Here's how the part is built. I have some questions about the finished solid (model axes, mm). A direction names the side the tool comes from. Coordinates: 2 decimals unless noted, no trailing zeros. Write each loop counter-clockwise with the first axis right and the second up, starting at its lowest first coordinate (ties: lowest second). Pieces come first, ordered by that corner, then holes. Notation, with made-up numbers: M -26.75,31 L -14.75,31 A32 ccw -14.75,60 Z; hole C -32,12 d9. An arc over 180 degrees is marked long. Use a Markdown table: item, result.
```python
from build123d import *

# Parameters (mm, degrees)
SKETCH1_W             = 10
SKETCH1_H             = 10.5
CUT_EXTRUDE1_DEPTH    = 11
CIRPATTERN1_COUNT     = 11
SKETCH3_R             = 12.5
BOSS_EXTRUDE1_DEPTH   = 10
CUT_EXTRUDE2_DEPTH    = 21
M2_TAPPED_HOLE1_D     = 1.6
M2_TAPPED_HOLE1_DEPTH = 9.8


with BuildPart() as part:
    # Sketch1 → Revolve1 (revolve)
    with BuildSketch(Plane(origin=(0, 0, 0), x_dir=(0, 0, -1), z_dir=(1, 0, 0))):
        with Locations((5, 5.25)):
            Rectangle(SKETCH1_W, SKETCH1_H)
    revolve(axis=Axis((0, 0, 0), (0, 0, -1)))

    # Sketch2 → Cut-Extrude1 (cut, through all)
    with BuildSketch(Plane.XY):
        with BuildLine():
            ThreePointArc((-0.824529961, 7.076123681), (0, 7.124), (0.824529961, 7.076123681))
            ThreePointArc((0.824529961, 7.076123681), (1.228997776, 8.871328839), (2.467796901, 10.232112622))
            ThreePointArc((2.467796901, 10.232112622), (0, 10.5255), (-2.467796901, 10.232112622))
            ThreePointArc((-2.467796901, 10.232112622), (-1.228997776, 8.871328839), (-0.824529961, 7.076123681))
        make_face()
    cut_extrude1 = extrude(amount=-CUT_EXTRUDE1_DEPTH, mode=Mode.SUBTRACT)

    # CirPattern1: Cut-Extrude1 ×11 about axis
    cirpattern1_axis = Axis((0, 0, 0), (0, 0, 1))
    for i in range(1, CIRPATTERN1_COUNT):
        add(cut_extrude1.rotate(cirpattern1_axis, i * 360 / CIRPATTERN1_COUNT), mode=Mode.SUBTRACT)

    # Sketch3 → Boss-Extrude1 (add)
    with BuildSketch(Plane.XY):
        Circle(SKETCH3_R)
    extrude(amount=BOSS_EXTRUDE1_DEPTH)

    # Sketch4 → Cut-Extrude2 (cut, through all)
    with BuildSketch(Plane.XY.offset(10)):
        with BuildLine():
            Line((2.7, 1.622498074), (2.7, -1.622498074))
            ThreePointArc((2.7, -1.622498074), (-3.15, 0), (2.7, 1.622498074))
        make_face()
    extrude(amount=-CUT_EXTRUDE2_DEPTH, mode=Mode.SUBTRACT)

    # M2 Tapped Hole1
    with Locations(Plane(origin=(12.5, 0, 0), x_dir=(0, 0, -1), z_dir=(1, 0, 0))):
        with Locations((-5, 0)):
            Hole(M2_TAPPED_HOLE1_D / 2, depth=M2_TAPPED_HOLE1_DEPTH)


solid = part.part
```
1. Will these pins go through, and if not, where does the flat tip stop? pin 1 Ø4 at (x, y) = (0, 0) entering from -Z; pin 2 Ø3 at (x, z) = (5, 7) entering from -Y; pin 3 Ø10 at (y, z) = (-9.5, 4) entering from -X; pin 4 Ø5 at (x, z) = (-8.5, 0.5) entering from +Y.
Answers follow:
| item | result |
|---|---|
| pin 1 | passes through |
| pin 2 | stops at y = -12 |
| pin 3 | stops at x = -11.66 |
| pin 4 | stops at y = 10.97 |
2. Suppose I cut it at C-C on z = 5. Write out the boundary of the cut face in (x, y).
Answers follow:
| item | result |
|---|---|
| outline | M 2.7,-1.62 A3.15 cw long 2.7,1.62 L 2.7,0.8 L 12.47,0.8 A12.5 ccw long 12.47,-0.8 L 2.7,-0.8 Z |
3. Suppose I cut it at B-B on y = -6. Write out the boundary of the cut face in (x, z).
Answers follow:
| item | result |
|---|---|
| outline | M -10.97,0 L -5.5,0 L -5.5,-10 L 5.5,-10 L 5.5,0 L 10.97,0 L 10.97,10 L -10.97,10 Z |
4. Which directions (+Z, -Z, +X, -X, +Y, -Y) give clear straight access to the entire face, cutting with the end or side of a thin tool? Please do faces 1 (the face through (9.55, -4.36, -5.07)), 2 (the face through (10.392, 1.502, -5.07)).
Answers follow:
| item | result |
|---|---|
| face 1 | -Z, +X, -Y |
| face 2 | -Z, +X, +Y |
5. We'd pull the mould along X, two halves only. Please class faces 3 (the face through (7.517, -4.883, -4.93)), 4 (the face through (11.923, 3.755, 4.93)), 5 (the face through (2.5, 2.3, -10)): +X half, -X half, draft (parallel to the pull), parting line (faces both ways), or undercut.
Answers follow:
| item | result |
|---|---|
| face 3 | undercut |
| face 4 | parting line |
| face 5 | draft |
6. I need wall thicknesses on probe 1 along Z at (x, y) = (8.5, 0); probe 2 along Y at (x, z) = (0, 2.5); probe 3 along X at (y, z) = (7.5, 6). Which ranges of each line are inside material? Lowest first, please.
Answers follow:
| item | result |
|---|---|
| probe 1 | z = -10 to 4.2, 5.8 to 10 |
| probe 2 | y = -12.5 to -3.15, 3.15 to 12.5 |
| probe 3 | x = -10 to 10 |
7. Suppose I cut it at A-A on x = 0. Write out the boundary of the cut face in (y, z).
Answers follow:
| item | result |
|---|---|
| outline | M -12.5,0 L -10.5,0 L -10.5,-10 L -3.15,-10 L -3.15,10 L -12.5,10 Z; M 3.15,-10 L 7.12,-10 L 7.12,0 L 12.5,0 L 12.5,10 L 3.15,10 Z |
